The listing builds one solid part. Answer for the finished solid, in the listing's coordinates (mm). Coordinates: 2 decimals unless noted, no trailing zeros. Write each loop counter-clockwise with the first axis right and the second up, starting at its lowest first coordinate (ties: lowest second). Pieces come first, ordered by that corner, then holes.
from build123d import *

# Parameters (mm, degrees)
F0_W     = 240
F0_H     = 190
F1_DEPTH = 1
F2_R     = 2
F3_T     = -1.6


with BuildPart() as f1:
    # F0 (on Front) → F1 (new body)
    with BuildSketch(Plane.XZ):
        Rectangle(F0_W, F0_H)
    extrude(amount=F1_DEPTH)

    # F2
    f2_edges = [f1.edges().sort_by_distance(p)[0] for p in [
        (120, -0.5, 95),
        (-120, -0.5, 95),
        (-120, -0.5, -95),
        (120, -0.5, -95),
    ]]
    fillet(f2_edges, radius=F2_R)

    # F3
    f3_openings = [f1.faces().sort_by_distance(p)[0] for p in [
        (0, 0, 0),
        (0, -1, 0),
    ]]
    offset(amount=F3_T, openings=f3_openings)


solid = f1.part
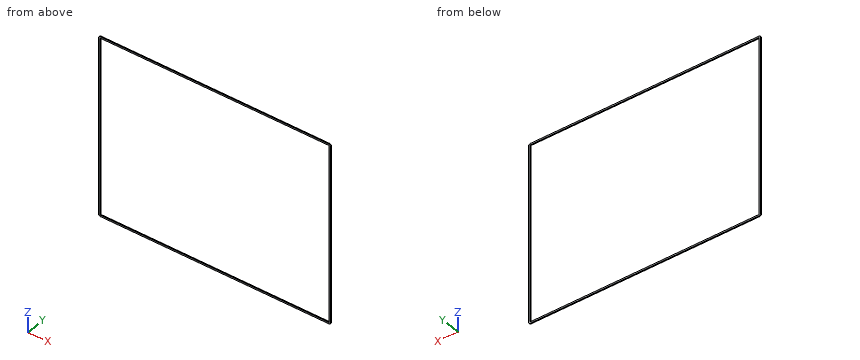
Q1. Find the intervals of material crossed by probe 1 along X at (y, z) = (-0.7, 56); probe 2 along Z at (x, y) = (74.5, -0.5), in increasing order.
Answers below:
probe 1: x = -120 to -118.4, 118.4 to 120
probe 2: z = -95 to -93.4, 93.4 to 95
Q2. The part is cut by section B-B, the plane x = -18.5. Write down the section's boundary in (y, z).
Answers below:
outline: (-1, -95) - (0, -95) - (0, -93.4) - (-1, -93.4) - close; (-1, 93.4) - (0, 93.4) - (0, 95) - (-1, 95) - close
Q3. The part is cut by section A-A, the plane z = -73.5. Write down the section's boundary in (x, y), then the cut area to 3 significant figures.
Answers below:
outline: (-120, -1) - (-118.4, -1) - (-118.4, 0) - (-120, 0) - close; (118.4, -1) - (120, -1) - (120, 0) - (118.4, 0) - close
area: 3.20 mm2
Q4. The part is cut by section C-C, the plane y = -0.8. Write down the section's boundary in (x, z), then the cut area to 3 significant figures.
Answers below:
outline: (-120, -93) arc R2 ccw to (-118, -95) - (118, -95) arc R2 ccw to (120, -93) - (120, 93) arc R2 ccw to (118, 95) - (-118, 95) arc R2 ccw to (-120, 93) - close; hole (-118.4, -93) arc R0.4 ccw to (-118, -93.4) - (118, -93.4) arc R0.4 ccw to (118.4, -93) - (118.4, 93) arc R0.4 ccw to (118, 93.4) - (-118, 93.4) arc R0.4 ccw to (-118.4, 93) - close
area: 1,360 mm2
